Source: CAD feature listing. Evaluate the final solid. Frame: model axes, mm. A direction names the side the tool comes from. Round coordinates to 2 decimals unless told otherwise and drop trailing zeros. Write each loop counter-clockwise with the first axis right and the second up, starting at its lowest first coordinate (ties: lowest second). Pieces come first, ordered by that corner, then holes. Notation, with made-up numbers: M 64.5,44 L 103.5,44 A8 ccw 103.5,56 Z; hole C -18.75,34 d8. An arc over 180 degrees is marked long. Answer in a Markdown table with one row per item. Add a question column.
Item 1: Contact query for flat-ended pins moving along their axis: pin 1 (0.5 mm diameter, centred on x = 58, z = 0.5, fed in from +Y); pin 2 (0.5 mm diameter, centred on x = -58.5, z = 0.5, fed in from +Y). Output: stop coordinate, or through.
Item 2: Mould query, pull axis X, two halves, no side actions, for faces 1 (the face through (-41.062, -40.252, 0.493)), 2 (the face through (-13.77, -61.99, 0.49)), 3 (the face through (-10, 57, 1)). Classes: released by +X, released by -X, zero draft, split by the parting line, or undercut.
Item 3: Cut plane C-C on z = 0.2. Return loops of the section in (x, y), and give its area (3 significant figures).
Item 4: Set-up query: faces 4 (the face through (-10, 57, 0)), 5 (the face through (-40.252, 41.062, 0.493)). Return all of +Z, -Z, +X, -X, +Y, -Y with unobstructed straight access to the full face (end or side cutting, diameter ignored); none if empty.
Item 5: Cut plane A-A on x = 0. Return loops of the section in (y, z), and give its area (3 significant figures).
Item 6: Material intervals for probe 1 along X at (y, z) = (-1, 0.15); probe 2 along X at (y, z) = (58.5, 0.3); probe 3 along Y at (x, z) = (50, 0.8), sorted ascending.
from build123d import *

# Parameters (mm, degrees)
F0_R     = 63.5
F0_R_2   = 57.5
F1_DEPTH = 1
F3_DEPTH = 25


with BuildPart() as f1:
    # F0 (on Top) → F1 (new body)
    with BuildSketch(Plane.XY):
        Circle(F0_R)
        Circle(F0_R_2, mode=Mode.SUBTRACT)
    extrude(amount=F1_DEPTH)

    # F2 (on Top) → F3 (cut)
    with BuildSketch(Plane.XY):
        Polygon((4.25, 60.75), (0, 60.75), (-4.25, 60.75), (-4.25, 56.5), (4.25, 56.5), align=None)
        Polygon((-4.25, -60.75), (0, -60.75), (4.25, -60.75), (4.25, -56.5), (-4.25, -56.5), align=None)
        Polygon((-60.75, 4.25), (-60.75, 0), (-60.75, -4.25), (-56.5, -4.25), (-56.5, 4.25), align=None)
        Polygon((60.75, -4.25), (60.75, 0), (60.75, 4.25), (56.5, 4.25), (56.5, -4.25), align=None)
    extrude(amount=F3_DEPTH, mode=Mode.SUBTRACT)


solid = f1.part
Results below:
| question | item | result |
|---|---|---|
| 1 | pin 1 | y = 26.4 |
| 1 | pin 2 | y = 25.28 |
| 2 | face 1 | undercut |
| 2 | face 2 | split by the parting line |
| 2 | face 3 | zero draft |
| 3 | outline | C 0,0 d127; hole M -60.75,-4.25 L -57.34,-4.25 A57.5 ccw -4.25,-57.34 L -4.25,-60.75 L 4.25,-60.75 L 4.25,-57.34 A57.5 ccw 57.34,-4.25 L 60.75,-4.25 L 60.75,4.25 L 57.34,4.25 A57.5 ccw 4.25,57.34 L 4.25,60.75 L -4.25,60.75 L -4.25,57.34 A57.5 ccw -57.34,4.25 L -60.75,4.25 Z |
| 3 | area | 2,170 mm2 |
| 4 | face 4 | -Z, +X, -X, +Y, -Y |
| 4 | face 5 | +Z, -Z |
| 5 | outline | M -63.5,0 L -60.75,0 L -60.75,1 L -63.5,1 Z; M 60.75,0 L 63.5,0 L 63.5,1 L 60.75,1 Z |
| 5 | area | 5.50 mm2 |
| 6 | probe 1 | -63.49 to -60.75, 60.75 to 63.49 |
| 6 | probe 2 | -24.7 to -4.25, 4.25 to 24.7 |
| 6 | probe 3 | -39.14 to -28.39, 28.39 to 39.14 |
